Here's how the part is built. I have some questions about the finished solid (model axes, mm). A direction names the side the tool comes from. Coordinates: 2 decimals unless noted, no trailing zeros. Write each loop counter-clockwise with the first axis right and the second up, starting at its lowest first coordinate (ties: lowest second). Pieces come first, ordered by that corner, then holes. Notation, with made-up numbers: (-21.75, 16) -> (-9.75, 16) arc R25 cw to (-9.75, 50) -> close; hole circle Ø2 at (-4, 27). An arc over 180 degrees is marked (long way). Use a Markdown table: item, result. Add a question column.
```python
from build123d import *

# Parameters (mm, degrees)
F1_DEPTH = 89
F3_DEPTH = 8.75
F4_T     = -2.5


# Not quite as in the source:
# - a shell that OpenCascade refuses in one call is made with other operations: the cavity is built on its own and cut out


with BuildPart() as f1:
    # F0 (on Top) → F1 (new body)
    with BuildSketch(Plane.XY):
        Polygon((50, 35.8578643763), (35.8578643763, 50), (-35.8578643763, 50), (-50, 35.8578643763), (-50, -35.8578643763), (-35.8578643763, -50), (35.8578643763, -50), (50, -35.8578643763), align=None)
    extrude(amount=-F1_DEPTH)

    # F2 (on face) → F3 (cut)
    with BuildSketch(Plane(origin=(0, 0, -89), x_dir=(1, 0, 0), z_dir=(0, 0, -1))):
        Polygon((-50, 35.8578643763), (-47.5, 34.8223305494), (-34.8223305494, 47.5), (-35.8578643763, 50), align=None)
        Polygon((-47.5, -34.8223304703), (-50, -35.8578643763), (-35.8578643763, -50), (-34.8223304703, -47.5), align=None)
        Polygon((50, 35.8578643763), (35.8578643763, 50), (34.8223305494, 47.5), (47.5, 34.8223305494), align=None)
        Polygon((34.8223305494, -47.5), (35.8578643763, -50), (50, -35.8578643763), (47.5, -34.8223305494), align=None)
    extrude(amount=-F3_DEPTH, mode=Mode.SUBTRACT)

    # F4: a shell. OpenCascade refuses it in one call, so the cavity is built on its own and cut out:
    # the body offset inwards by the wall thickness, plus a prism from it out through each open face.
    f4_core = offset(f1.part, amount=F4_T, kind=Kind.INTERSECTION, mode=Mode.PRIVATE)
    f4_exits = [f4_core.faces().sort_by_distance(p)[0] for p in [
        (0, 0, -86.5),
    ]]
    add(f4_core, mode=Mode.SUBTRACT)
    extrude(f4_exits, amount=-F4_T, mode=Mode.SUBTRACT)


solid = f1.part
```
Q1. Suppose I cut it at A-A, the plane z = -30.5. Write out the boundary of the cut face in (x, y).
Q2. Please list where these lines run through material, in increasing order: line 1 (X direction, y = 30, z = -53.5); line 2 (Z direction, x = 29, y = 31).
Q3. Which directions (+Z, -Z, +X, -X, +Y, -Y) give clear straight access to the entire face, cutting with the end or side of a thin tool? Please do faces 4 (the flat face through (39.499, -39.288, -83.296)), 5 (the flat face through (-41.07, 41.25, -39.6)), 6 (the flat face through (-43.03, -42.83, -39.56)).
Q4. Suppose I cut it at D-D, the plane y = 38.5. Write out the boundary of the cut face in (x, z).
Q5. Suppose I cut it at B-B, the plane x = -16. Write out the boundary of the cut face in (y, z).
Q6. Thinking about a two-plate mould opening in Z: for faces 1 (the flat face through (41.25, 41.07, -39.6)), 2 (the flat face through (-42, 42, -80.25)), 3 (the flat face through (-1, -50, -44)), which applies, released by +Z, released by -Z, zero draft, split by the parting line, or undercut?
Q7. Will these pins go through, and if not, where does the flat tip stop? pin 1 (4.5 mm diameter, centred on x = 42.5, y = 44, fed in from -Z); pin 2 (5 mm diameter, centred on x = 29, y = -27, fed in from -Z).
Answer key:
| question | item | result |
|---|---|---|
| 1 | outline | (-50, -35.86) -> (-35.86, -50) -> (35.86, -50) -> (50, -35.86) -> (50, 35.86) -> (35.86, 50) -> (-35.86, 50) -> (-50, 35.86) -> close; hole (-47.5, -34.82) -> (-34.82, -47.5) -> (34.82, -47.5) -> (47.5, -34.82) -> (47.5, 34.82) -> (34.82, 47.5) -> (-34.82, 47.5) -> (-47.5, 34.82) -> close |
| 2 | line 1 | x = -50 to -47.5, 47.5 to 50 |
| 2 | line 2 | z = -2.5 to 0 |
| 3 | face 4 | -Z |
| 3 | face 5 | none |
| 3 | face 6 | +Z, -Z, -X, -Y |
| 4 | outline | (-47.36, -80.25) -> (-43.82, -80.25) -> (-43.82, -89) -> (-40.29, -89) -> (-40.29, -77.75) -> (-43.82, -77.75) -> (-43.82, -2.5) -> (43.82, -2.5) -> (43.82, -77.75) -> (40.29, -77.75) -> (40.29, -89) -> (43.82, -89) -> (43.82, -80.25) -> (47.36, -80.25) -> (47.36, 0) -> (-47.36, 0) -> close |
| 5 | outline | (-50, -89) -> (-47.5, -89) -> (-47.5, -2.5) -> (47.5, -2.5) -> (47.5, -89) -> (50, -89) -> (50, 0) -> (-50, 0) -> close |
| 6 | face 1 | undercut |
| 6 | face 2 | released by -Z |
| 6 | face 3 | zero draft |
| 7 | pin 1 | stops at z = -80.25 |
| 7 | pin 2 | stops at z = -2.5 |
